The listing builds one solid part. Answer for the finished solid, in the listing's coordinates (mm). Face numbers are marked on the shaded views. A direction names the side the tool comes from. Round coordinates to 2 decimals unless told otherwise and drop trailing zeros. Write each loop counter-clockwise with the first axis right and the second up, starting at its lowest first coordinate (ties: lowest second). Pieces come first, ordered by that corner, then holes. Notation, with made-up numbers: (-33, -25) - (-2, -25) arc R9 ccw to (-2, -12) - close; hole circle Ø1 at (62.25, 86.5). An arc over 180 degrees is marked (long way). Answer as CSV lines item,"result". Start each with the question number.
Item 1: A cutting plane is placed at B-B on x = 11.5. Determine the outline of the cut face in (y, z).
Item 2: A cutting plane is placed at A-A on y = 12.5. Determine the outline of the cut face in (x, z).
Item 3: Which of the six approach directions +Z, -Z, +X, -X, +Y, -Y give full straight-line access (tool end or side, diameter ignored) to the marked faces 1, 2, 3 and 4?
Item 4: Straight lines are drawn through the part: line 1 along Y through (x, z) = (-2.4, 0); line 2 along Y through (x, z) = (-9, 0.5); line 3 along X through (y, z) = (-14, -5). For each, find the intervals that lie inside material, in ascending order. Write a range as [from, to].
Item 5: Flat-ended cylindrical pins translate along their axes: pin 1 (12 mm diameter, centred on x = 9.5, y = 14.5, fed in from -Z); pin 2 (5 mm diameter, centred on y = -12.5, z = 0, fed in from +X); pin 3 (10 mm diameter, centred on x = 7.5, y = 43.5, fed in from -Z); pin 4 (6 mm diameter, centred on x = -9.5, z = -5, fed in from +Y). Find the tip coordinate at first contact, or state that the pin passes through.
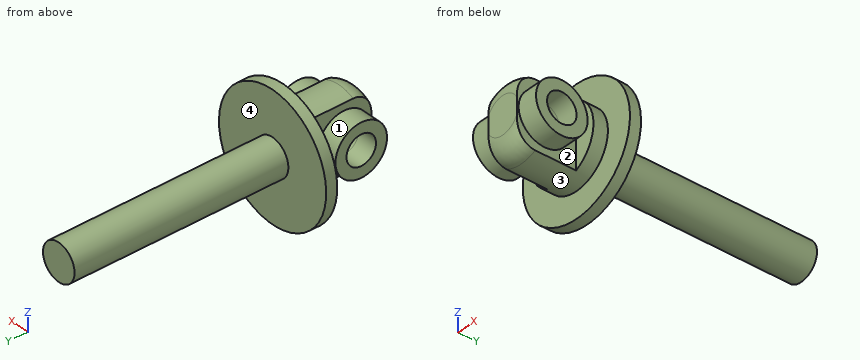
```python
from build123d import *
from build123d.topology import SkipClean

# Parameters (mm, degrees)
SKETCH1_R           = 17
BOSS_EXTRUDE1_DEPTH = 3
SKETCH2_R           = 5
BOSS_EXTRUDE2_DEPTH = 58
SKETCH3_R           = 10
BOSS_EXTRUDE3_DEPTH = 20
FILLET1_R           = 5
CUT_EXTRUDE1_START  = -8.930286
SKETCH4_W           = 7.220401321
SKETCH4_H           = 16.086512415
CUT_EXTRUDE1_DEPTH  = 17.860572
SKETCH5_R           = 4
CUT_EXTRUDE2_DEPTH  = 20
SKETCH6_R           = 7
SKETCH6_R_2         = 4
BOSS_EXTRUDE4_DEPTH = 10


with BuildPart() as part:
    # Sketch1 → Boss-Extrude1 (new body)
    with BuildSketch(Plane(origin=(0, 0, 0), x_dir=(1, 0, 0), z_dir=(0, 1, 0))):
        with Locations(Location((0, 0, 0), (0, 0, 270))):
            Circle(SKETCH1_R)
    extrude(amount=BOSS_EXTRUDE1_DEPTH)

    # Sketch2 → Boss-Extrude2 (add)
    with BuildSketch(Plane(origin=(0, 3, 0), x_dir=(1, 0, 0), z_dir=(0, 1, 0))):
        with Locations(Location((0, 0, 0), (0, 0, 90))):
            Circle(SKETCH2_R)
    extrude(amount=BOSS_EXTRUDE2_DEPTH)

    # Sketch3 → Boss-Extrude3 (add)
    with BuildSketch(Plane.XZ):
        with Locations(Location((0, 0, 0), (0, 0, 90))):
            Circle(SKETCH3_R)
    extrude(amount=BOSS_EXTRUDE3_DEPTH)

    # Fillet1
    fillet1_edges = [part.edges().sort_by_distance(p)[0] for p in [
        (0, -20, -10),
    ]]
    fillet(fillet1_edges, radius=FILLET1_R)

    # Sketch4 → Cut-Extrude1 (cut)
    with BuildSketch(Plane.XY.offset(CUT_EXTRUDE1_START)):
        with Locations((8.110200661, -11.956743792)):
            Rectangle(SKETCH4_W, SKETCH4_H)
        with Locations((-8.110200661, -11.956743792)):
            Rectangle(SKETCH4_W, SKETCH4_H)
    extrude(amount=CUT_EXTRUDE1_DEPTH, mode=Mode.SUBTRACT)

    # Sketch5 → Cut-Extrude2 (cut)
    with BuildSketch(Plane(origin=(4.5, 0, 0), x_dir=(0, 0, -1), z_dir=(1, 0, 0))):
        with Locations(Location((0, -12.5, 0), (0, 0, 90))):
            Circle(SKETCH5_R)
    extrude(amount=-CUT_EXTRUDE2_DEPTH, mode=Mode.SUBTRACT)

    # Sketch6 → Boss-Extrude4 (add, symmetric)
    with SkipClean():  # the faces are left unmerged after this step: merging them gives an invalid solid
        with BuildSketch(Plane(origin=(0, 0, 0), x_dir=(0, 0, -1), z_dir=(1, 0, 0))):
            with Locations(Location((0, -12.5, 0), (0, 0, 90))):
                Circle(SKETCH6_R)
            with Locations((0, -12.5)):
                Circle(SKETCH6_R_2, mode=Mode.SUBTRACT)
        extrude(amount=BOSS_EXTRUDE4_DEPTH, both=True)


solid = part.part
```
Geometry says:
1,outline,"(0, -12.52) - (3, -12.52) - (3, 12.52) - (0, 12.52) - close"
2,outline,"circle Ø10 at (0, 0)"
3,face 1,"-X"
3,face 2,"+X"
3,face 3,"none"
3,face 4,"+Y"
4,line 1,"y = [-20, -16.5], [-8.5, 61]"
4,line 2,"y = [-19.48, -16.47], [-8.53, -5.52], [-3.91, 3]"
4,line 3,"x = [-10, 10]"
5,pin 1,"stops at z = -3.57"
5,pin 2,"passes through"
5,pin 3,"stops at z = -4.33"
5,pin 4,"stops at y = 3"
